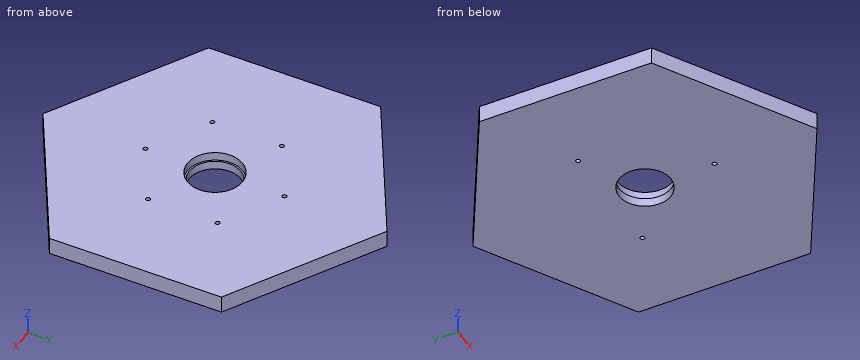
```python
from build123d import *

# Parameters (mm, degrees)
PAD002_DEPTH            = 10
SKETCH009_R             = 15.975
POCKET007_DEPTH         = 5
SKETCH008_R             = 15
POCKET008_DEPTH         = 5
SKETCH024_R             = 1.25
HOLE004_DEPTH           = 10.001
SKETCH066_R             = 1.25
HOLE005_DEPTH           = 6.248924
HOLE005_TIPS_R          = 1.25
BODY002_PLACEMENT_ANGLE = 180


with BuildPart() as part:
    # Sketch007 → Pad002 (new body)
    with BuildSketch(Plane.XY):
        Polygon((86.60254, 50), (0, 100), (-86.60254, 50), (-86.60254, -50), (0, -100), (86.60254, -50), align=None)
    extrude(amount=PAD002_DEPTH)

    # Sketch009 → Pocket007 (cut)
    with BuildSketch(Plane(origin=(0, 0, 0), x_dir=(1, 0, 0), z_dir=(0, 0, -1))):
        Circle(SKETCH009_R)
    extrude(amount=-POCKET007_DEPTH, mode=Mode.SUBTRACT)

    # Sketch008 → Pocket008 (cut)
    with BuildSketch(Plane.XY.offset(10)):
        Circle(SKETCH008_R)
    extrude(amount=-POCKET008_DEPTH, mode=Mode.SUBTRACT)

    # Sketch024 → Hole004 (cut, through all)
    with BuildSketch(Plane.XY.offset(10)):
        with Locations((35, -20.207259)):
            Circle(SKETCH024_R)
        with Locations((0, 40.414519)):
            Circle(SKETCH024_R)
        with Locations((-35, -20.207259)):
            Circle(SKETCH024_R)
    extrude(amount=-HOLE004_DEPTH, mode=Mode.SUBTRACT)

    # Sketch066 (on Face4 of Hole004) → Hole005 (cut)
    with BuildSketch(Plane(origin=(0, 0, 0), x_dir=(1, 0, 0), z_dir=(0, 0, -1))):
        with Locations((35, -20.207259)):
            Circle(SKETCH066_R)
        with Locations((0, 40.414519)):
            Circle(SKETCH066_R)
        with Locations((-35, -20.207259)):
            Circle(SKETCH066_R)
    extrude(amount=-HOLE005_DEPTH, mode=Mode.SUBTRACT)

    # Hole005 tips → Hole005 tip 1 section 0
    with BuildSketch(Plane(origin=(0, 0, 6.248924), x_dir=(1, 0, 0), z_dir=(0, 0, -1)), mode=Mode.PRIVATE) as hole005_tip_1_s0:
        with Locations((35, -20.207259)):
            Circle(HOLE005_TIPS_R)
    loft([hole005_tip_1_s0.sketch, Vertex(35, 20.207259, 7)], mode=Mode.SUBTRACT)

    # Hole005 tips → Hole005 tip 2 section 0
    with BuildSketch(Plane(origin=(0, 0, 6.248924), x_dir=(1, 0, 0), z_dir=(0, 0, -1)), mode=Mode.PRIVATE) as hole005_tip_2_s0:
        with Locations((0, 40.414519)):
            Circle(HOLE005_TIPS_R)
    loft([hole005_tip_2_s0.sketch, Vertex(0, -40.414519, 7)], mode=Mode.SUBTRACT)

    # Hole005 tips → Hole005 tip 3 section 0
    with BuildSketch(Plane(origin=(0, 0, 6.248924), x_dir=(1, 0, 0), z_dir=(0, 0, -1)), mode=Mode.PRIVATE) as hole005_tip_3_s0:
        with Locations((-35, -20.207259)):
            Circle(HOLE005_TIPS_R)
    loft([hole005_tip_3_s0.sketch, Vertex(-35, 20.207259, 7)], mode=Mode.SUBTRACT)


with BuildPart() as part_1:
    # Body002 placement: moved
    add(part.part.moved(Location((3.1, 54.8, 93.3))).rotate(Axis((3.1, 54.8, 93.3), (1, 0, 0)), BODY002_PLACEMENT_ANGLE))


solid = part_1.part
```
Here's how the part is built. I have some questions about the finished solid (model axes, mm). Round coordinates to 2 decimals unless told otherwise and drop trailing zeros. Loops run counter-clockwise (first coordinate to the right, second up) from the corner with the lowest first, then second, coordinate; pieces in that order, holes last. Notation, with made-up numbers: (45.5, -14.75) -> (65.5, -14.75) arc R4 cw to (65.5, -9.75) -> close; hole circle Ø7 at (-14.5, 16.25). An arc over 180 degrees is marked (long way). Answer as CSV lines item,"result". Start each with the question number.
1. Imagine slicing it at C-C on y = -10. Write out the boundary of the cut face in (x, z).
2. Imagine slicing it at A-A on y = 54.8. Write out the boundary of the cut face in (x, z) (3 decimals), plus the area to 3 significant figures.
3. Imagine slicing it at D-D on x = 33.5. Write out the boundary of the cut face in (y, z), plus the area to 3 significant figures.
4. I need wall thicknesses on probe 1 along X at (y, z) = (34.5, 89.75); probe 2 along Y at (x, z) = (3.1, 91.2) (3 decimals); probe 3 along Y at (x, z) = (-31.9, 92.25). Which ranges of each line are inside material? Lowest first, please. Write a range as from..to.
5. I'm going to push flat-ended pins straight in: P1, Ø1.5, axis at x = -60, z = 91, coming from the -Y side; P2, Ø2, axis at x = 70, z = 85, coming from the -Y side; P3, Ø6, axis at x = 29.5, z = 89.5, coming from the +Y side. Where does each tip first touch, or does it pass through?
6. Imagine slicing it at B-B on z = 90.25. Write out the boundary of the cut face in (x, y) (3 decimals).
Solution:
1,outline,"(-57.87, 83.3) -> (64.07, 83.3) -> (64.07, 93.3) -> (-57.87, 93.3) -> close"
2,outline,"(-83.503, 83.3) -> (-11.9, 83.3) -> (-11.9, 88.3) -> (-12.875, 88.3) -> (-12.875, 93.3) -> (-83.503, 93.3) -> close; (18.1, 83.3) -> (89.703, 83.3) -> (89.703, 93.3) -> (19.075, 93.3) -> (19.075, 88.3) -> (18.1, 88.3) -> close"
2,area,"1,420 mm²"
3,outline,"(-27.65, 83.3) -> (137.25, 83.3) -> (137.25, 93.3) -> (-27.65, 93.3) -> close"
3,area,"1,650 mm²"
4,probe 1,"-83.5..-33.15, -30.65..36.85, 39.35..89.7"
4,probe 2,"-45.2..13.135, 15.635..38.825, 70.775..93.965, 96.465..154.8"
4,probe 3,"-24.99..33.34, 35.84..73.76, 76.26..134.59"
5,P1,"y = -9.2"
5,P2,"y = -7.15"
5,P3,"y = 141.29"
6,outline,"(-83.503, 4.8) -> (3.1, -45.2) -> (89.703, 4.8) -> (89.703, 104.8) -> (3.1, 154.8) -> (-83.503, 104.8) -> close; hole circle Ø2.5 at (-31.9, 34.593); hole circle Ø2.5 at (-31.9, 75.007); hole circle Ø31.95 at (3.1, 54.8); hole circle Ø2.5 at (3.1, 14.385); hole circle Ø2.5 at (3.1, 95.215); hole circle Ø2.5 at (38.1, 34.593); hole circle Ø2.5 at (38.1, 75.007)"
